Design review of the part shown in the three views and the two pictorial views. Dimensions are in mm from the part's minimum x, y and z. A direction names the side the tool comes from. Coordinates: 2 decimals unless noted, no trailing zeros. Write each loop counter-clockwise with the first axis right and the second up, starting at its lowest first coordinate (ties: lowest second). Pieces come first, ordered by that corner, then holes. Notation, with made-up numbers: (23.25, 9.5) - (80.25, 9.5) arc R37 ccw to (80.25, 45.5) - close; hole circle Ø9 at (-11, 85). An arc over 180 degrees is marked (long way). Answer as CSV lines item,"result". Start each with the question number.
Q1. Machinability: for the marked faces 4, 5 and 6, which of the approach directions +Z, -Z, +X, -X, +Y, -Y give a long, thin tool a straight path to every point of the face, cutting with its end or side? Answer none if there is none.
Q2. We need section A-A (z = 9). Write out the cut boundary in (x, y), plus the area to 3 significant figures.
Q3. For line 1 along X through (y, z) = (1, 9); line 2 along Y through (x, z) = (30.5, 2.25); line 3 along X through (y, z) = (20.5, 1), list the stretches that pass through material, from the lowest coordinate up. Write a range as [from, to].
Q4. We need section D-D (y = 34.85). Write out the cut boundary in (x, z).
Q5. We need section B-B (x = 23.5). Write out the cut boundary in (y, z), plus the area to 3 significant figures.
Q6. We need section C-C (z = 2.25). Write out the cut boundary in (x, y), plus the area to 3 significant figures.
Q7. Clearance check with flat-ended pins moving along their axes: pin 1 (1.5 mm diameter, centred on x = 10.5, z = 4.5, fed in from +Y); pin 2 (1.5 mm diameter, centred on x = 21.5, y = 11.5, fed in from +Z). State where each tip first meets the part, or that it passes through.
Q8. Mouldability with a two-part tool opening along X and no side actions: class the marked faces 1, 2 and 3 as pulls with the +X half, pulls with the -X half, needs draft (parallel to the pull), parting line crosses it, or undercut.
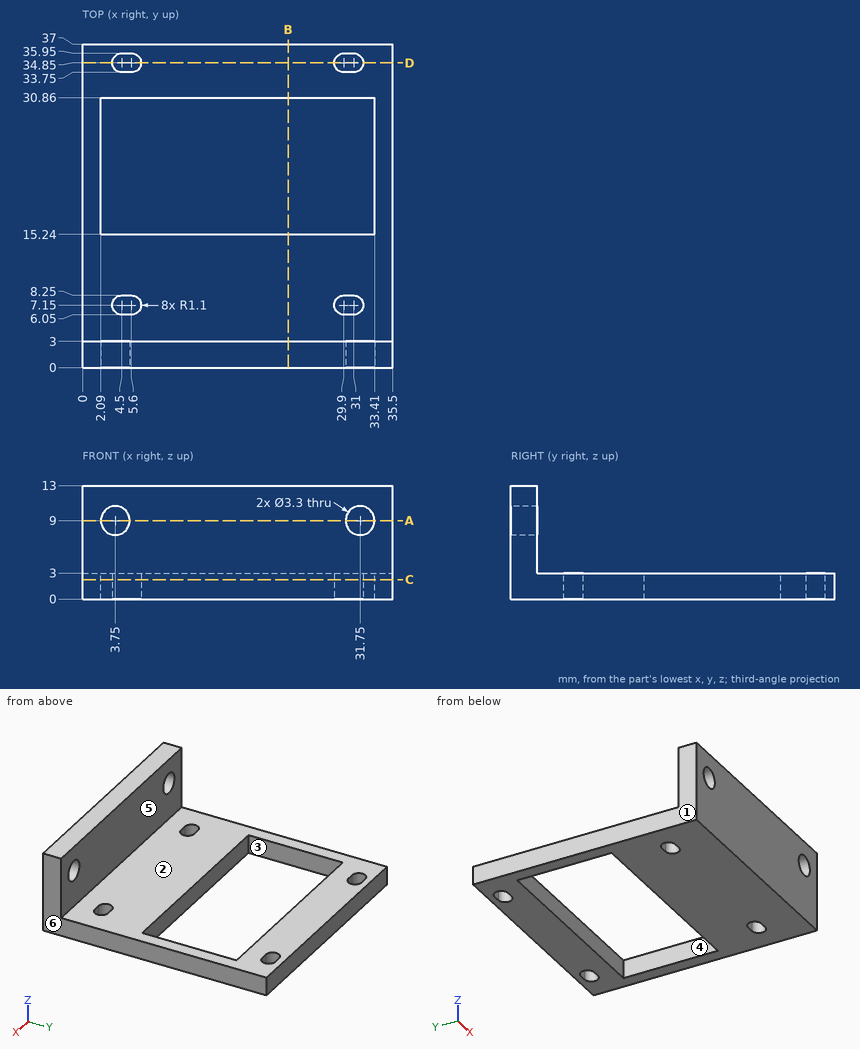
Results list:
1,face 4,"+Z, -Z"
1,face 5,"+Z, +X, -X, +Y"
1,face 6,"+Z, -Z, +X, +Y, -Y"
2,outline,"(0, 0) - (2.1, 0) - (2.1, 3) - (0, 3) - close; (5.4, 0) - (30.1, 0) - (30.1, 3) - (5.4, 3) - close; (33.4, 0) - (35.5, 0) - (35.5, 3) - (33.4, 3) - close"
2,area,"86.7 mm2"
3,line 1,"x = [0, 2.1], [5.4, 30.1], [33.4, 35.5]"
3,line 2,"y = [0, 6.05], [8.25, 15.24], [30.86, 33.75], [35.95, 37]"
3,line 3,"x = [0, 2.09], [33.41, 35.5]"
4,outline,"(0, 0) - (3.4, 0) - (3.4, 3) - (0, 3) - close; (6.7, 0) - (28.8, 0) - (28.8, 3) - (6.7, 3) - close; (32.1, 0) - (35.5, 0) - (35.5, 3) - (32.1, 3) - close"
5,outline,"(0, 0) - (15.24, 0) - (15.24, 3) - (3, 3) - (3, 13) - (0, 13) - close; (30.86, 0) - (37, 0) - (37, 3) - (30.86, 3) - close"
5,area,"94.1 mm2"
6,outline,"(0, 0) - (35.5, 0) - (35.5, 37) - (0, 37) - close; hole (2.09, 15.24) - (33.41, 15.24) - (33.41, 30.86) - (2.09, 30.86) - close; hole (4.5, 6.05) - (5.6, 6.05) arc R1.1 ccw to (5.6, 8.25) - (4.5, 8.25) arc R1.1 ccw to start; hole (4.5, 33.75) - (5.6, 33.75) arc R1.1 ccw to (5.6, 35.95) - (4.5, 35.95) arc R1.1 ccw to start; hole (29.9, 6.05) - (31, 6.05) arc R1.1 ccw to (31, 8.25) - (29.9, 8.25) arc R1.1 ccw to start; hole (29.9, 33.75) - (31, 33.75) arc R1.1 ccw to (31, 35.95) - (29.9, 35.95) arc R1.1 ccw to start"
6,area,"799 mm2"
7,pin 1,"stops at y = 3"
7,pin 2,"stops at z = 3"
8,face 1,"pulls with the -X half"
8,face 2,"needs draft"
8,face 3,"undercut"
